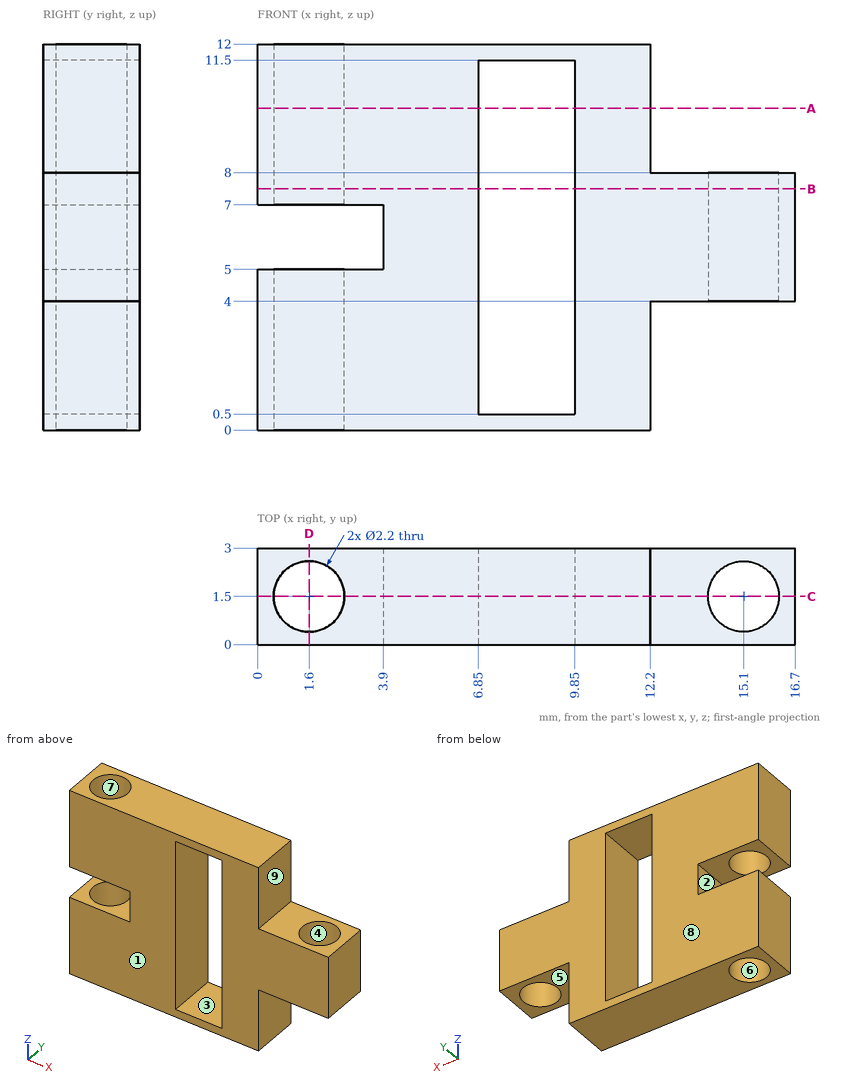
For this review, use the dimensioned drawing (mm, ordinates from the lowest corner) and the shaded views. A direction names the side the tool comes from. Give positions to 0.01 mm unless a question says otherwise; leave off trailing zeros. Loops run counter-clockwise (first coordinate to the right, second up) from the corner with the lowest first, then second, coordinate; pieces in that order, holes last.
Item 1: Tool access review of the marked faces 1, 2, 3, 4 and 5: name each direction out of +Z, -Z, +X, -X, +Y, -Y from which nothing blocks a thin tool from reaching the whole face with its end or side.
Item 2: For line 1 along X through (y, z) = (1.5, 3.7); line 2 along X through (y, z) = (1.5, 5.65); line 3 along X through (y, z) = (1.5, 4.9), list the stretches that pass through material, from the lowest coordinate up.
Item 3: Take a section at C-C, the plane y = 1.5. State the section outline as (x, z) points, and give its area (3 significant figures).
Item 4: Take a section at A-A, the plane z = 10. State the section outline as (x, y) points.
Item 5: Insertion check: pin 1 (1 mm diameter, centred on x = 14, z = 10.5, fed in from -Y); pin 2 (1.5 mm diameter, centred on x = 14.5, y = 1.5, fed in from -Z); pin 3 (1.6 mm diameter, centred on y = 1, z = 6, fed in from -X); pin 4 (1.5 mm diameter, centred on x = 15.5, y = 2, fed in from +Z). Each pin has a flat end and moves straight along its axis. Give the tip position at first contact, or say it passes through.
Item 6: Draft analysis for pull direction Y (two halves, no side actions). For the marked faces 6, 7, 8 and 9, state which applies: +Y half, -Y half, draft (parallel to the pull), parting line (faces both ways), or undercut.
Item 7: Take a section at D-D, the plane x = 1.6. State the section outline as (y, z) points, and give its area (3 significant figures).
Item 8: Take a section at B-B, the plane z = 7.5. State the section outline as (x, y) points.
Calculated:
1. face 1: +Z, -Z, +X, -X, -Y
1. face 2: -X, +Y, -Y
1. face 3: +Y, -Y
1. face 4: +Z, -Z
1. face 5: -Z, +X, +Y, -Y
2. line 1: x = 0 to 0.5, 2.7 to 6.85, 9.85 to 12.2
2. line 2: x = 3.9 to 6.85, 9.85 to 14, 16.2 to 16.7
2. line 3: x = 0 to 0.5, 2.7 to 6.85, 9.85 to 14, 16.2 to 16.7
3. outline: (0, 0) - (0.5, 0) - (0.5, 5) - (0, 5) - close; (0, 7) - (0.5, 7) - (0.5, 12) - (0, 12) - close; (2.7, 0) - (12.2, 0) - (12.2, 4) - (14, 4) - (14, 8) - (12.2, 8) - (12.2, 12) - (2.7, 12) - (2.7, 7) - (3.9, 7) - (3.9, 5) - (2.7, 5) - close; (16.2, 4) - (16.7, 4) - (16.7, 8) - (16.2, 8) - close; hole (6.85, 0.5) - (9.85, 0.5) - (9.85, 11.5) - (6.85, 11.5) - close
3. area: 92.8 mm2
4. outline: (0, 0) - (6.85, 0) - (6.85, 3) - (0, 3) - close; (9.85, 0) - (12.2, 0) - (12.2, 3) - (9.85, 3) - close; hole circle Ø2.2 at (1.6, 1.5)
5. pin 1: passes through
5. pin 2: stops at z = 4
5. pin 3: stops at x = 3.9
5. pin 4: stops at z = 8
6. face 6: undercut
6. face 7: undercut
6. face 8: +Y half
6. face 9: draft
7. outline: (0, 0) - (0.4, 0) - (0.4, 5) - (0, 5) - close; (0, 7) - (0.4, 7) - (0.4, 12) - (0, 12) - close; (2.6, 0) - (3, 0) - (3, 5) - (2.6, 5) - close; (2.6, 7) - (3, 7) - (3, 12) - (2.6, 12) - close
7. area: 8.00 mm2
8. outline: (0, 0) - (6.85, 0) - (6.85, 3) - (0, 3) - close; (9.85, 0) - (16.7, 0) - (16.7, 3) - (9.85, 3) - close; hole circle Ø2.2 at (1.6, 1.5); hole circle Ø2.2 at (15.1, 1.5)
